Autodesk Inventor part; units mm, degrees
ref_plane "YZ Plane" through (0, 0, 0) normal (1, 0, 0) x (0, 1, 0)
ref_plane "XZ Plane" through (0, 0, 0) normal (0, 1, 0) x (-1, 0, 0)
ref_plane "XY Plane" through (0, 0, 0) normal (0, 0, 1) x (1, 0, 0)
sketch "Эскиз1" plane through (0, 0, 0) normal (0, 0, 1) x (1, 0, 0)
  line L0 (0, 0) -> (-28.3405, 0)
  line L1 (-28.3405, 0) -> (-28.3405, 3)
  line L2 (-28.3405, 3) -> (0, 3)
  line L3 (0, 3) -> (0, 0)
  line L4 (-28.3405, 0) -> (-26.0995, 0)
  line L5 (-26.0995, 0) -> (-26.0995, 18)
  line L6 (-26.0995, 18) -> (-28.3405, 18)
  line L7 (-28.3405, 18) -> (-28.3405, 0)
  line L8 (0, -3.6) -> (0, 21.6)
  point P0 (-26.0995, 3)
  dimension "d0" = 28.3405
  dimension "d1" = 3
  dimension "d2" = 2.241
  dimension "d3" = 18
revolve "Вращение1" add sketch "Эскиз1" angle 360 about axis through (0, -10, 0) along (0, 1, 0)
sketch "Эскиз2" plane through (0, 3, 0) normal (0, 1, 0) x (1, 0, 0)
  line L0 (0, 10) -> (0, -10) construction
  line L1 (-5, 10) -> (-5, -10)
  line L2 (5, -10) -> (5, 10)
  arc A0 (5, 10) -> (-5, 10) centre (0, 10) ccw
  arc A1 (-5, -10) -> (5, -10) centre (0, -10) ccw
  circle A2 centre (8.1, 0) radius 2.1
  circle A3 centre (-8.1, 0) radius 2.1
  point P0 (0, 0)
  dimension "d5" = 10
  dimension "d6" = 10
  dimension "d7" = 4.2
  dimension "d8" = 3.1
extrude "Выдавливание1" cut sketch "Эскиз2" against normal blind 10
chamfer "Фаска1" distance 2.2 angle 45 1 edges at (-10.2, 3, 0)
chamfer "Фаска2" distance 2.2 angle 45 1 edges at (6, 3, 0)
properties part number "кроватка"
Check sheet for the modelled part. Datum: model origin and axes. Units: mm. A direction names the side the tool comes from. Coordinates: 2 decimals unless noted, no trailing zeros. Write each loop counter-clockwise with the first axis right and the second up, starting at its lowest first coordinate (ties: lowest second). Pieces come first, ordered by that corner, then holes. Notation, with made-up numbers: M -29,18.5 L -7,18.5 A8 ccw -7,23.5 Z; hole C 84.5,62 d1. An arc over 180 degrees is marked long. Use one line per item in the form item = value.
Item 1: Sectioned sample at A-A, the plane z = 0. Record the cut outline in (x, y), and give its area (3 significant figures).
Answer below:
outline = M -28.34,0 L -10.2,0 L -10.2,0.8 L -12.4,3 L -26.1,3 L -26.1,18 L -28.34,18 Z; M -6,0 L -5,0 L -5,1.8 L -6,0.8 Z; M 5,0 L 6,0 L 6,0.8 L 5,1.8 Z; M 10.2,0 L 28.34,0 L 28.34,18 L 26.1,18 L 26.1,3 L 12.4,3 L 10.2,0.8 Z
area = 174 mm^2
Item 2: Sectioned sample at C-C, the plane y = 7.75. Record the cut outline in (x, z).
Answer below:
outline = C 0,0 d56.68; hole C 0,0 d52.2
Item 3: Release check for a two-part mould opening along X. For faces 4 (the face through (6.144, 9.126, -27.667)), 5 (the face through (-6, 0, -6)), 6 (the face through (0, 2, -15)) record: pulls with the +X half, pulls with the -X half, needs draft (parallel to the pull), parting line crosses it, or undercut.
Answer below:
face_4 = parting line crosses it
face_5 = needs draft
face_6 = undercut
Item 4: Sectioned sample at D-D, the plane x = -21.5. Record the cut outline in (y, z), and give its area (3 significant figures).
Answer below:
outline = M 0,-18.46 L 18,-18.46 L 18,-14.8 L 3,-14.8 L 3,14.8 L 18,14.8 L 18,18.46 L 0,18.46 Z
area = 221 mm^2
Item 5: Material ranges on L1, parallel to Z at x = 0, y = 13.5; L2, parallel to Y at x = 23.5, z = -6; L3, parallel to X at y = 8.75, z = 11, recorded low to high. Write a range as from..to.
Answer below:
L1 = -28.34..-26.1, 26.1..28.34
L2 = 0..3
L3 = -26.12..-23.67, 23.67..26.12
Item 6: Sectioned sample at B-B, the plane z = 14. Record the cut outline in (x, y), and give its area (3 significant figures).
Answer below:
outline = M -24.64,0 L -3,0 L -3,3 L -22.03,3 L -22.03,18 L -24.64,18 Z; M 3,0 L 24.64,0 L 24.64,18 L 22.03,18 L 22.03,3 L 3,3 Z
area = 208 mm^2
Item 7: Set-up check for faces 1 (the face through (-24.894, 10.605, 7.84)), 2 (the face through (5, 1.5, 0.1)), 3 (the face through (-25.1, 18, -8.3)): record each of +Z, -Z, +X, -X, +Y, -Y from which the full face is reachable in a straight line by a thin tool's end or side.
Answer below:
face_1 = +Y
face_2 = +Y, -Y
face_3 = +Z, -Z, +X, -X, +Y
Item 8: Gauge pin test, flat ends, axial feed: pin 1 Ø15.5 at (x, z) = (-3, 2) entering from +Y; pin 2 Ø10 at (y, z) = (13, -20.5) entering from -X; pin 3 Ø1 at (x, y) = (-15, 13) entering from +Z; pin 4 Ø3.5 at (x, z) = (-8.1, 0) entering from -Y. Record the tip position at first contact, or that the pin passes through.
Answer below:
pin_1 = 3
pin_2 = -23.73
pin_3 = 24.35
pin_4 = through
